Geometry: see drawing. Coordinates: mm, zero at the bounding-box minimum. A direction names the side the tool comes from. Give positions to 0.01 mm unless a question says otherwise; leave off trailing zeros. Write each loop counter-clockwise with the first axis right and the second up, starting at its lowest first coordinate (ties: lowest second). Pieces come first, ordered by that corner, then holes. Notation, with made-up numbers: (-16, -26) - (11, -26) arc R28 cw to (11, -5) - close; hole circle Ø8 at (12, 30.5). An arc over 180 degrees is marked (long way). Use a Markdown table: item, result. Add a question column.
1. Section query C-C, the plane x = 13. Return loops of the section in (y, z).
2. Section query A-A, the plane y = 18. Return loops of the section in (x, z).
3. Section query B-B, the plane z = 11. Return loops of the section in (x, y).
4. Section query D-D, the plane x = 3.5. Return loops of the section in (y, z).
5. Pin query (flat end, axial travel): pin 1 (9 mm diameter, centred on x = 14, z = 24.5, fed in from +Y); pin 2 (8 mm diameter, centred on x = 14.5, y = 23, fed in from +Z). Return the tip coordinate at first contact, or that it passes through.
6. Material intervals for probe 1 along Y at (x, z) = (13, 1); probe 2 along Z at (x, y) = (42, 29.5), sorted ascending.
7. Set-up query: the marked faces 1 and 2. Return all of +Z, -Z, +X, -X, +Y, -Y with unobstructed straight access to the full face (end or side cutting, diameter ignored); none if empty.
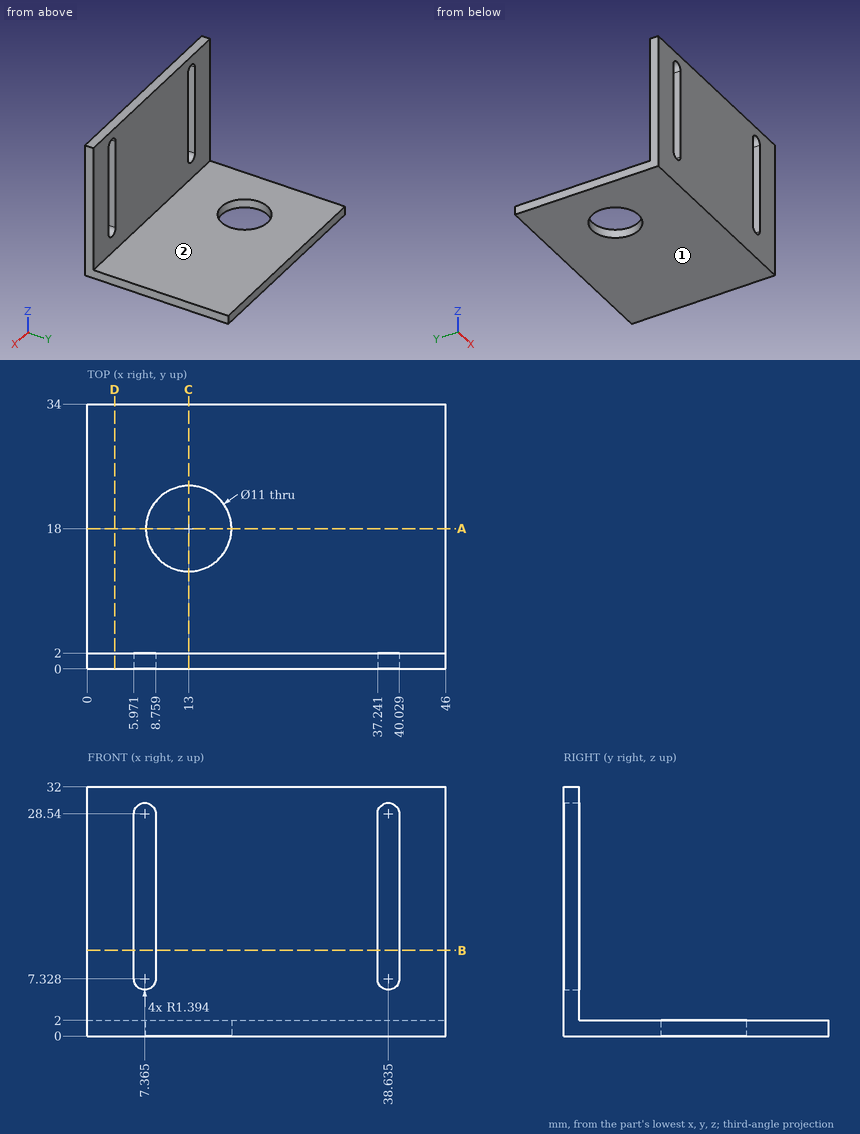
Result sheet:
| question | item | result |
|---|---|---|
| 1 | outline | (0, 0) - (12.5, 0) - (12.5, 2) - (2, 2) - (2, 32) - (0, 32) - close; (23.5, 0) - (34, 0) - (34, 2) - (23.5, 2) - close |
| 2 | outline | (0, 0) - (7.5, 0) - (7.5, 2) - (0, 2) - close; (18.5, 0) - (46, 0) - (46, 2) - (18.5, 2) - close |
| 3 | outline | (0, 0) - (5.97, 0) - (5.97, 2) - (0, 2) - close; (8.76, 0) - (37.24, 0) - (37.24, 2) - (8.76, 2) - close; (40.03, 0) - (46, 0) - (46, 2) - (40.03, 2) - close |
| 4 | outline | (0, 0) - (34, 0) - (34, 2) - (2, 2) - (2, 32) - (0, 32) - close |
| 5 | pin 1 | stops at y = 2 |
| 5 | pin 2 | stops at z = 2 |
| 6 | probe 1 | y = 0 to 12.5, 23.5 to 34 |
| 6 | probe 2 | z = 0 to 2 |
| 7 | face 1 | -Z, +X, -X, +Y, -Y |
| 7 | face 2 | +Z, +X, -X, +Y |
